from build123d import *

# Parameters (mm, degrees)
SKETCH_1_W      = 25
SKETCH_1_H      = 24
SKETCH_1_R      = 1.1
EXTRUDE_1_DEPTH = 1
SKETCH_2_W      = 22
SKETCH_2_H      = 6
EXTRUDE_2_DEPTH = 2
SKETCH_3_W      = 9
SKETCH_3_H      = 9
EXTRUDE_3_DEPTH = 2.5
SKETCH_4_R      = 3.5
EXTRUDE_4_DEPTH = 1.5
SKETCH_5_W      = 7
SKETCH_5_H      = 7
EXTRUDE_5_DEPTH = 1


with BuildPart() as part:
    # 草图1 → 凸台-拉伸1 (new body)
    with BuildSketch(Plane.XY):
        Rectangle(SKETCH_1_W, SKETCH_1_H)
        with Locations((-10.5, 10)):
            Circle(SKETCH_1_R, mode=Mode.SUBTRACT)
        with Locations((-10.5, -3)):
            Circle(SKETCH_1_R, mode=Mode.SUBTRACT)
        with Locations((10.5, -3)):
            Circle(SKETCH_1_R, mode=Mode.SUBTRACT)
        with Locations((10.5, 10)):
            Circle(SKETCH_1_R, mode=Mode.SUBTRACT)
    extrude(amount=EXTRUDE_1_DEPTH)

    # 草图2 → 凸台-拉伸2 (add)
    with BuildSketch(Plane.XY.offset(1)):
        with Locations((0, -9)):
            Rectangle(SKETCH_2_W, SKETCH_2_H)
    extrude(amount=EXTRUDE_2_DEPTH)

    # 草图3 → 凸台-拉伸3 (add)
    with BuildSketch(Plane(origin=(0, 0, 0), x_dir=(-1, 0, 0), z_dir=(0, 0, -1))):
        with Locations((0, -2.5)):
            Rectangle(SKETCH_3_W, SKETCH_3_H)
    extrude(amount=EXTRUDE_3_DEPTH)

    # 草图4 → 凸台-拉伸4 (add)
    with BuildSketch(Plane(origin=(0, 0, -2.5), x_dir=(-1, 0, 0), z_dir=(0, 0, -1))):
        with Locations((0, -2.5)):
            Circle(SKETCH_4_R)
    extrude(amount=EXTRUDE_4_DEPTH)

    # 草图5 → 凸台-拉伸5 (add)
    with BuildSketch(Plane(origin=(0, 0, 0), x_dir=(-1, 0, 0), z_dir=(0, 0, -1))):
        with Locations((0, 5.5)):
            Rectangle(SKETCH_5_W, SKETCH_5_H)
    extrude(amount=EXTRUDE_5_DEPTH)


solid = part.part
Here's how the part is built. I have some questions about the finished solid (model axes, mm). A direction names the side the tool comes from. Give positions to 0.01 mm unless a question says otherwise; leave off trailing zeros. Order: outer loops, then holes, each group sorted by start corner. A loop starts at its lowest first (then second) coordinate and runs counter-clockwise, first axis right, second up. Notation, with made-up numbers: M 7,10.5 L 14,10.5 A21 cw 14,22.5 Z; hole C -29.75,-33.75 d9. An arc over 180 degrees is marked long. Answer as a JSON object with one key per item and string values. Group by question number.
1) On a 3-axis mill with a long thin cutter (end or side, diameter ignored), from which of +Z, -Z, +X, -X, +Y, -Y can I reach the whole of each face in a straight line? I mean faces 4 (the flat face through (-3.5, 5.5, -0.5)), 5 (the flat face through (0, -7, -1)), 6 (the flat face through (3, 0, -2.5)), 7 (the flat face through (4.5, -3, -1)). Say none if no direction works.
2) Please list where these lines run through material, in increasing order: L1, parallel to Y at x = 10.5, z = 0.75; L2, parallel to Z at x = 0.75, y = -8.5; L3, parallel to Y at x = 1, z = -0.25. Write a range as [from, to].
3) I'm going to push flat-ended pins straight in: pin 1 Ø0.8 at (x, z) = (1, -1.5) entering from +Y; pin 2 Ø0.5 at (y, z) = (6, -0.5) entering from -X; pin 3 Ø0.8 at (x, z) = (1, -1.5) entering from -Y. Where does each tip first touch, or does it pass through?
4) Suppose I cut it at C-C, the plane y = 3.25. Write out the boundary of the cut face in (x, z), plus the area to 3 significant figures.
5) Suppose I cut it at A-A, the plane x = -10.5. Write out the boundary of the cut face in (y, z), plus the area to 3 significant figures.
6) Suppose I cut it at D-D, the plane y = 10. Write out the boundary of the cut face in (x, z).
7) We'd pull the mould along Y, two halves only. Please class faces 1 (the cylindrical face through (11.516, -3.421, 0.493)), 2 (the flat face through (0, 9, -0.5)), 3 (the flat face through (-4.5, -3, -1)): pulls with the +Y half, pulls with the -Y half, needs draft (parallel to the pull), parting line crosses it, or undercut.
8) Suppose I cut it at B-B, the plane z = 0.5. Write out the boundary of the cut face in (x, y), plus the area to 3 significant figures.
Results found:
{
 "1": {"face 4": "-Z, -X, +Y", "face 5": "-Z, +X, -X, -Y", "face 6": "-Z", "face 7": "-Z, +X, +Y, -Y"},
 "2": {"L1": "[-12, -4.1], [-1.9, 8.9], [11.1, 12]", "L2": "[0, 3]", "L3": "[-7, 9]"},
 "3": {"pin 1": "y = 2", "pin 2": "x = -3.5", "pin 3": "y = -7"},
 "4": {"outline": "M -12.5,0 L -3.5,0 L -3.5,-1 L 3.5,-1 L 3.5,0 L 12.5,0 L 12.5,1 L -12.5,1 Z", "area": "32.0 mm²"},
 "5": {"outline": "M -12,0 L -4.1,0 L -4.1,1 L -6,1 L -6,3 L -12,3 Z; M -1.9,0 L 8.9,0 L 8.9,1 L -1.9,1 Z; M 11.1,0 L 12,0 L 12,1 L 11.1,1 Z", "area": "31.6 mm²"},
 "6": {"outline": "M -12.5,0 L -11.6,0 L -11.6,1 L -12.5,1 Z; M -9.4,0 L 9.4,0 L 9.4,1 L -9.4,1 Z; M 11.6,0 L 12.5,0 L 12.5,1 L 11.6,1 Z"},
 "7": {"face 1": "undercut", "face 2": "pulls with the +Y half", "face 3": "needs draft"},
 "8": {"outline": "M -12.5,-12 L 12.5,-12 L 12.5,12 L -12.5,12 Z; hole C -10.5,-3 d2.2; hole C -10.5,10 d2.2; hole C 10.5,-3 d2.2; hole C 10.5,10 d2.2", "area": "585 mm²"}
}
